Check sheet for the drawn part. Datum: minimum x, y, z corner. Units: mm. A direction names the side the tool comes from. Coordinates: 2 decimals unless noted, no trailing zeros. Order: outer loops, then holes, each group sorted by start corner. A loop starts at its lowest first (then second) coordinate and runs counter-clockwise, first axis right, second up. Notation, with made-up numbers: (-19.5, 51) - (30.5, 51) arc R29 ccw to (30.5, 88) - close; hole circle Ø3 at (29, 38.25). An arc over 180 degrees is marked (long way). One line per item, written item: value. Start each with the question number.
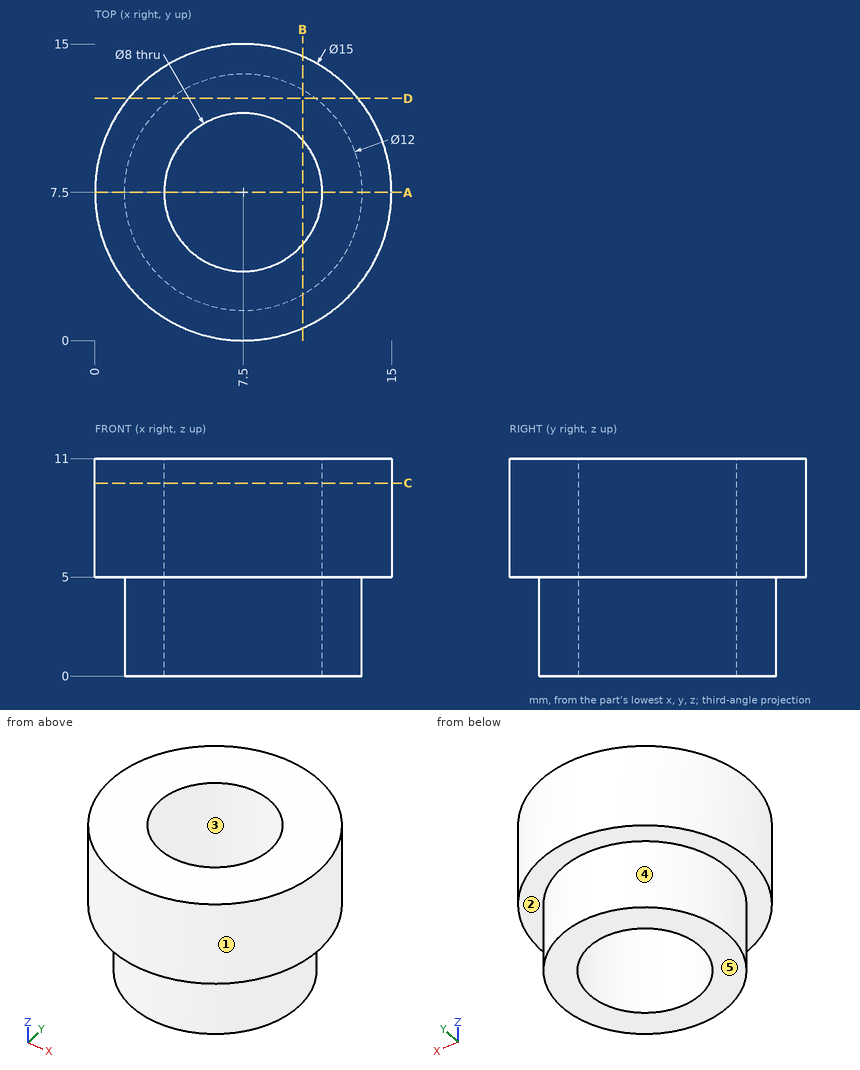
Q1. Release check for a two-part mould opening along X. For the marked faces 3, 4 and 5 record: released by +X, released by -X, zero draft, split by the parting line, or undercut.
Q2. Cross-section at A-A, the plane y = 7.5. Enter the section's corners in (x, z), and give its area (3 significant figures).
Q3. Cross-section at D-D, the plane y = 12.25. Enter the section's corners in (x, z).
Q4. Gauge pin test, flat ends, axial feed: P1, Ø6, axis at x = 4, z = 4, coming from the +Y side; P2, Ø1, axis at x = 10, y = 7, coming from the +Z side; P3, Ø3, axis at x = 2, z = 9, coming from the -Y side; P4, Ø7.5, axis at x = 4, y = 5, coming from the -Z side. Record the tip position at first contact, or that the pin passes through.
Q5. Cross-section at C-C, the plane z = 9.75. Enter the section's corners in (x, y), and give its area (3 significant figures).
Q6. Cross-section at B-B, the plane x = 10.5. Enter the section's corners in (y, z), and give its area (3 significant figures).
Q7. Set-up check for the marked faces 1 and 2: record each of +Z, -Z, +X, -X, +Y, -Y from which the full face is reachable in a straight line by a thin tool's end or side.
Q8. Material ranges on probe 1 along Y at (x, z) = (7.5, 8); probe 2 along Y at (x, z) = (7.5, 4); probe 3 along Z at (x, y) = (11.5, 1.5), recorded low to high.
Check result:
1. face 3: undercut
1. face 4: split by the parting line
1. face 5: zero draft
2. outline: (0, 5) - (1.5, 5) - (1.5, 0) - (3.5, 0) - (3.5, 11) - (0, 11) - close; (11.5, 0) - (13.5, 0) - (13.5, 5) - (15, 5) - (15, 11) - (11.5, 11) - close
2. area: 62.0 mm2
3. outline: (1.7, 5) - (3.83, 5) - (3.83, 0) - (11.17, 0) - (11.17, 5) - (13.3, 5) - (13.3, 11) - (1.7, 11) - close
4. P1: stops at y = 14.97
4. P2: passes through
4. P3: stops at y = 1.16
4. P4: stops at z = 0
5. outline: circle Ø15 at (7.5, 7.5); hole circle Ø8 at (7.5, 7.5)
5. area: 126 mm2
6. outline: (0.63, 5) - (2.3, 5) - (2.3, 0) - (4.85, 0) - (4.85, 11) - (0.63, 11) - close; (10.15, 0) - (12.7, 0) - (12.7, 5) - (14.37, 5) - (14.37, 11) - (10.15, 11) - close
6. area: 76.2 mm2
7. face 1: +Z, -Z
7. face 2: -Z
8. probe 1: y = 0 to 3.5, 11.5 to 15
8. probe 2: y = 1.5 to 3.5, 11.5 to 13.5
8. probe 3: z = 5 to 11
